from build123d import *

# Parameters (mm, degrees)
F0_W      = 110
F0_H      = 77
F1_DEPTH  = 33.5
F2_W      = 100
F2_H      = 23.5
F4_DEPTH  = 72
F3_W      = 2
F3_H      = 8.335
F5_DEPTH  = 40
F6_W      = 76
F6_H      = 60
F7_DEPTH  = 20.9
F8_W      = 47
F8_H      = 5
F9_DEPTH  = 17
F10_W     = 47
F10_H     = 10
F11_DEPTH = 2
F13_DEPTH = 55.8
F14_SIZE  = 5


with BuildPart() as f1:
    # F0 (on Top) → F1 (new body)
    with BuildSketch(Plane.XY):
        Rectangle(F0_W, F0_H)
    extrude(amount=F1_DEPTH)

    # F2 (on face) → F4 (cut)
    with BuildSketch(Plane(origin=(0, 38.5, 0), x_dir=(-1, 0, 0), z_dir=(0, 1, 0))):
        with Locations((0, 16.75)):
            Rectangle(F2_W, F2_H)
    extrude(amount=-F4_DEPTH, mode=Mode.SUBTRACT)

    # F3 (on face) → F5 (join)
    with BuildSketch(Plane(origin=(0, 38.5, 0), x_dir=(-1, 0, 0), z_dir=(0, 1, 0))):
        with Locations((49, 16.4975)):
            Rectangle(F3_W, F3_H)
        with Locations((-49, 16.4975)):
            Rectangle(F3_W, F3_H)
    extrude(amount=-F5_DEPTH)

    # F6 (on face) → F7 (cut)
    with BuildSketch(Plane.XY.offset(33.5)):
        with Locations((0, 8.5)):
            Rectangle(F6_W, F6_H)
    extrude(amount=-F7_DEPTH, mode=Mode.SUBTRACT)

    # F8 (on face) → F9 (join)
    with BuildSketch(Plane(origin=(0, 38.5, 0), x_dir=(-1, 0, 0), z_dir=(0, 1, 0))):
        with Locations((0, 2.5)):
            Rectangle(F8_W, F8_H)
    extrude(amount=F9_DEPTH)

    # F10 (on face) → F11 (join)
    with BuildSketch(Plane.XY.offset(5)):
        with Locations((0, 50.5)):
            Rectangle(F10_W, F10_H)
    extrude(amount=F11_DEPTH)

    # F12 (on face) → F13 (cut)
    with BuildSketch(Plane(origin=(-23.5, 0, 0), x_dir=(0, -1, 0), z_dir=(-1, 0, 0))):
        Polygon((-55.5, 7), (-55.5, 5), (-45.5, 7), align=None)
    extrude(amount=-F13_DEPTH, mode=Mode.SUBTRACT)

    # F14
    f14_edges = [f1.edges().sort_by_distance(p)[0] for p in [
        (55, -38.5, 16.75),
        (-55, -38.5, 16.75),
    ]]
    chamfer(f14_edges, length=F14_SIZE)


solid = f1.part
Model file for the job. Use its own axes, mm. A direction names the side the tool comes from. Round coordinates to 2 decimals unless told otherwise and drop trailing zeros. Order: outer loops, then holes, each group sorted by start corner. A loop starts at its lowest first (then second) coordinate and runs counter-clockwise, first axis right, second up. Notation, with made-up numbers: M 82.5,-33.75 L 96.5,-33.75 A18 cw 96.5,-6.75 Z; hole C -2,-12.5 d7. An arc over 180 degrees is marked long. Write each question's results on one line, items separated by ' | '. Start each with the question number.
(1) Saw through at A-A, the plane y = -16. Give the cut face in (x, z), then the cut area to 3 significant figures.
(2) Probe probe 1 along X at (y, z) = (9.5, 22.5); probe 2 along X at (y, z) = (37, 16.5); probe 3 along Z at (x, y) = (-10, -28). List the from-to ranges inside material, lowest first. Write a range as from..to.
(3) Two-plate mould, pull along X, no slides. Class faces 1 (the face through (1, -33.5, 17)), 2 (the face through (55, 2, 17)), 3 (the face through (-55, 2, 17)): pulls with the +X half, pulls with the -X half, needs draft (parallel to the pull), parting line crosses it, or undercut.
(4) Saw through at D-D, the plane x = 27. Give the cut face in (y, z), then the cut area to 4 significant figures.
(5) Which spindle directions (+Z, -Z, +X, -X, +Y, -Y) get a long thin tool onto all of the face, cutting with end or side? Do faces 4 (the face through (-38, 8, 31)), 5 (the face through (23.5, 47, 3)), 6 (the face through (1, 7, 5)), 7 (the face through (-23.5, 47, 3)). Say none if no direction does.
(6) Saw through at B-B, the plane x = -42. Give the cut face in (y, z).
(7) Drop flat-ended pins along their axis: pin 1 (7 mm diameter, centred on x = 1.5, z = 19.5, fed in from +Y); pin 2 (3.5 mm diameter, centred on y = 43, z = 5, fed in from +X); pin 3 (4 mm diameter, centred on x = -43.5, z = 27, fed in from +Y). Give the stop position or say it passes through.
(8) Saw through at C-C, the plane z = 14. Give the cut face in (x, y), then the cut area to 4 significant figures.
Established:
1) outline: M -55,0 L 55,0 L 55,33.5 L 38,33.5 L 38,28.5 L 50,28.5 L 50,5 L -50,5 L -50,28.5 L -38,28.5 L -38,33.5 L -55,33.5 Z | area: 955 mm^2
2) probe 1: x = -55..-50, 50..55 | probe 2: x = -55..-48, 48..55 | probe 3: z = 0..5, 28.5..33.5
3) face 1: undercut | face 2: pulls with the +X half | face 3: pulls with the -X half
4) outline: M -38.5,0 L 38.5,0 L 38.5,5 L -33.5,5 L -33.5,28.5 L -21.5,28.5 L -21.5,33.5 L -38.5,33.5 Z | area: 587.5 mm^2
5) face 4: +Z, +Y | face 5: +Z, -Z, +X, +Y | face 6: none | face 7: +Z, -Z, -X, +Y
6) outline: M -38.5,0 L 38.5,0 L 38.5,5 L -33.5,5 L -33.5,28.5 L 38.5,28.5 L 38.5,33.5 L -38.5,33.5 Z
7) pin 1: stops at y = -33.5 | pin 2: stops at x = 23.5 | pin 3: stops at y = 38.5
8) outline: M -55,-33.5 L -50,-38.5 L 50,-38.5 L 55,-33.5 L 55,38.5 L 48,38.5 L 48,-1.5 L 50,-1.5 L 50,-33.5 L -50,-33.5 L -50,-1.5 L -48,-1.5 L -48,38.5 L -55,38.5 Z | area: 1,405 mm^2
